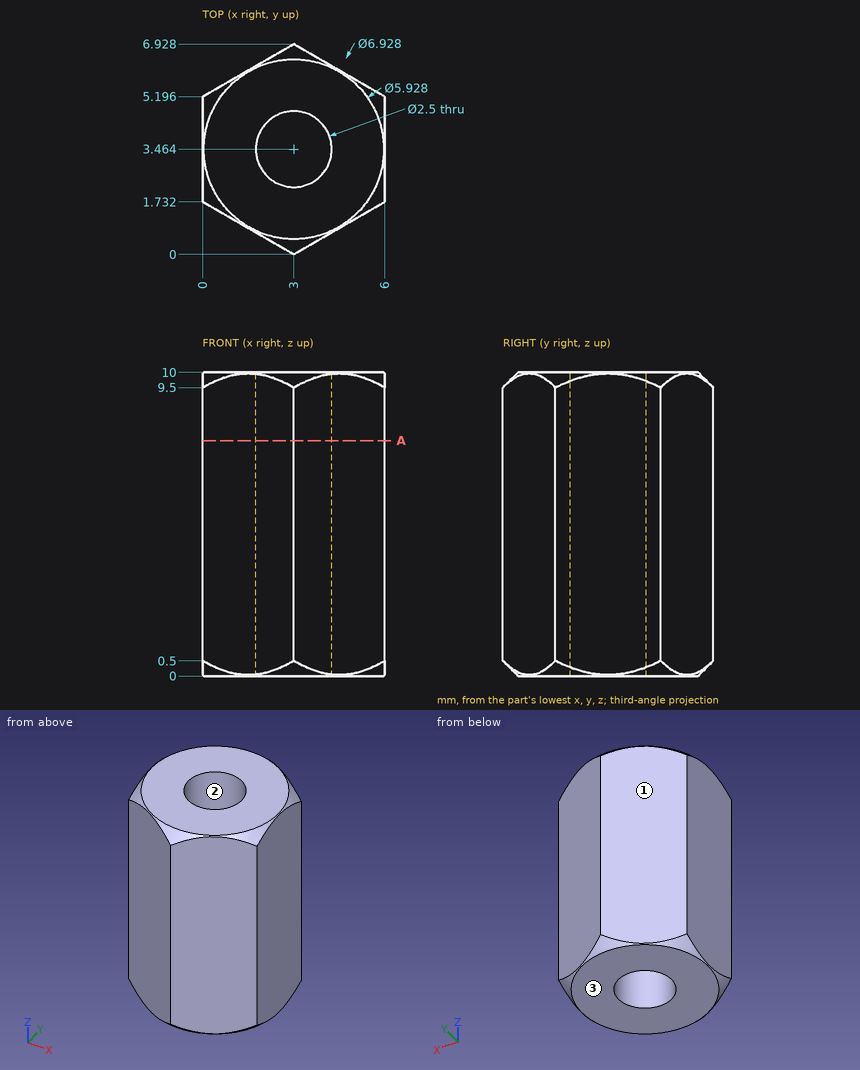
Here's the drawing with two shaded views (mm, measured from the low corner). I have some questions. Coordinates: 2 decimals unless noted, no trailing zeros. Loops run counter-clockwise (first coordinate to the right, second up) from the corner with the lowest first, then second, coordinate; pieces in that order, holes last. Notation, with made-up numbers: (43.5, 60.25) -> (86.5, 60.25) arc R13 cw to (86.5, 80.25) -> close; hole circle Ø1 at (58, 28.25). An arc over 180 degrees is marked (long way). Use one line per item in the form item = value. Start each with the question number.
(1) If we section it at A-A (z = 7.75): Please give me the cut outline in (x, y), then the cut area to 3 significant figures.
(2) Will this pin go through, and if not, where does the flat tip stop? pin 1 (1.5 mm diameter, centred on x = 3, y = 3.46, fed in from +Z) (3 decimals).
(3) Please list where these lines run through material, in increasing order: line 1 along X through (y, z) = (3.25, 1.5); line 2 along Y through (x, z) = (4.1, 6.5) (1 decimal); line 3 along X through (y, z) = (4, 6.5).
(4) We'd pull the mould along Y, two halves only. Please class the marked faces 1, 2 and 3: pulls with the +Y half, pulls with the -Y half, needs draft (parallel to the pull), parting line crosses it, or undercut.
Verdict:
q1.outline = (0, 1.73) -> (3, 0) -> (6, 1.73) -> (6, 5.2) -> (3, 6.93) -> (0, 5.2) -> close; hole circle Ø2.5 at (3, 3.46)
q1.area = 26.3 mm²
q2.pin_1 = through
q3.line_1 = 0 to 1.77, 4.23 to 6
q3.line_2 = 0.6 to 2.9, 4.1 to 6.3
q3.line_3 = 0 to 1.87, 4.13 to 6
q4.face_1 = pulls with the +Y half
q4.face_2 = undercut
q4.face_3 = needs draft
